Source: three-view drawing plus pictorial views. Frame: mm from the lowest corner of the part. Give positions to 0.01 mm unless a question says otherwise; leave off trailing zeros. Order: outer loops, then holes, each group sorted by start corner. A loop starts at its lowest first (then second) coordinate and runs counter-clockwise, first axis right, second up. Notation, with made-up numbers: M 1,71.5 L 14,71.5 A15 cw 14,85.5 Z; hole C 19.5,-20.5 d7. An arc over 180 degrees is marked long. Use CSV: the item, a comma, the result in double quotes. Start each with the question number.
Item 1: Section query B-B on y = 1.7. Return loops of the section in (x, z), and give its area (3 significant figures).
Item 2: Section query A-A on x = 7. Return loops of the section in (y, z).
Item 3: Ray query, probe 1 along X at (y, z) = (1.8, 6); probe 2 along Z at (x, y) = (30.5, 0.6) (1 decimal); probe 3 along X at (y, z) = (4.05, 13) (1 decimal). Return the intervals inside material, ascending. Write a range as from..to.
Item 4: Pull-direction query (Z, two-part tool) for the marked faces 1, 2 and 3; classes: +Z half, -Z half, draft (parallel to the pull), parting line (faces both ways), or undercut.
Item 5: Section query C-C on x = 18. Return loops of the section in (y, z), and give its area (3 significant figures).
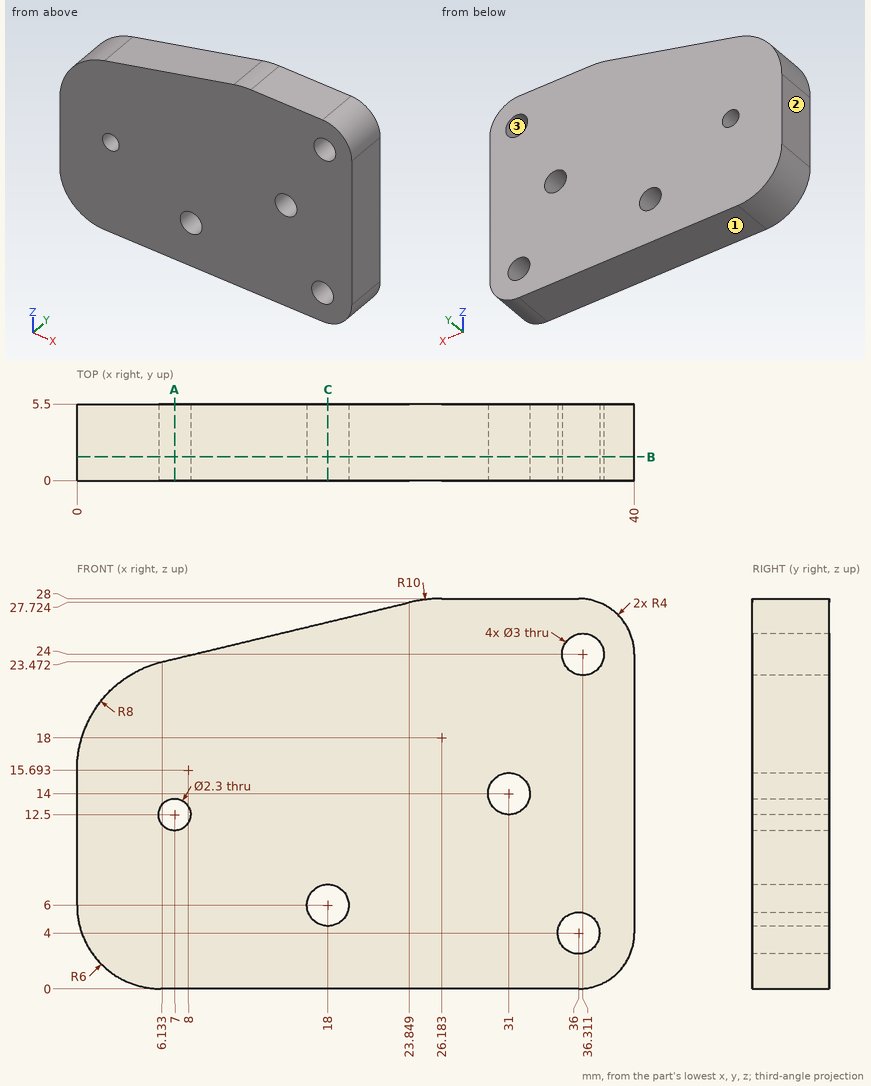
Verdict:
1,outline,"M 0,6 A6 ccw 6,0 L 36,0 A4 ccw 40,4 L 40,24 A4 ccw 36,28 L 26.18,28 A10 ccw 23.85,27.72 L 6.13,23.47 A8 ccw 0,15.69 Z; hole C 7,12.5 d2.3; hole C 18,6 d3; hole C 31,14 d3; hole C 36,4 d3; hole C 36.31,24 d3"
1,area,"990 mm2"
2,outline,"M 0,0 L 5.5,0 L 5.5,11.35 L 0,11.35 Z; M 0,13.65 L 5.5,13.65 L 5.5,23.68 L 0,23.68 Z"
3,probe 1,"0..16.5, 19.5..40"
3,probe 2,"0..12.6, 15.4..28"
3,probe 3,"0..6, 8..29.9, 32.1..40"
4,face 1,"-Z half"
4,face 2,"draft"
4,face 3,"undercut"
5,outline,"M 0,0 L 5.5,0 L 5.5,4.5 L 0,4.5 Z; M 0,7.5 L 5.5,7.5 L 5.5,26.32 L 0,26.32 Z"
5,area,"128 mm2"
